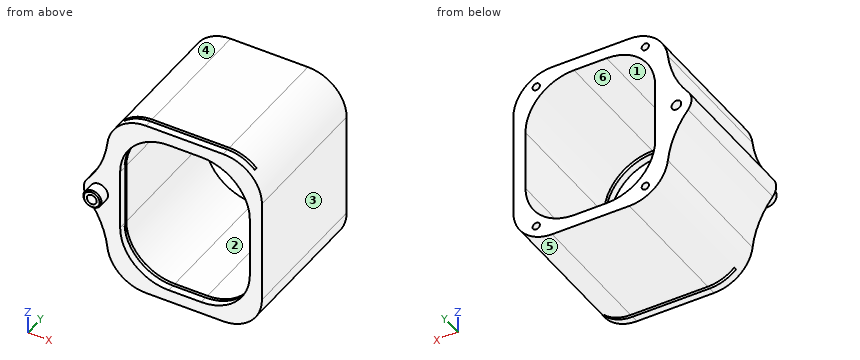
from build123d import *

# Parameters (mm, degrees)
CUT_EXTRUDE1_REACH       = 130.224
SKETCH3_W                = 13.598117377
SKETCH3_H                = 26.0138757
BOSS_EXTRUDE1_DEPTH      = 75
BOSS_EXTRUDE1_DEPTH_BACK = 75
SKETCH2_W                = 127
SKETCH2_H                = 117
BOSS_EXTRUDE3_START      = -117
BOSS_EXTRUDE3_DEPTH      = 117
CUT_EXTRUDE2_DEPTH       = 200.610245228
CUT_EXTRUDE2_DEPTH_BACK  = 200.610245228
SKETCH5_W                = 107
SKETCH5_H                = 130
CUT_EXTRUDE3_DEPTH       = 239.158035766
CUT_EXTRUDE3_DEPTH_BACK  = 239.158035766
SKETCH6_W                = 108
SKETCH6_H                = 2.5
FILLET3_R                = 40
FILLET2_R                = 32
CHAMFER1_SIZE            = 1
SKETCH7_R                = 3
CUT_EXTRUDE4_DEPTH       = 8


with BuildPart() as part:
    # Sketch1 → Revolve1 (revolve)
    with BuildSketch(Plane.XY, mode=Mode.PRIVATE) as revolve1_sk:
        Polygon((4, 0), (4, 127), (12.5, 127), (12.5, 10), (7.5, 10), (7.5, 0), align=None)
    revolve(revolve1_sk.sketch.rotate(Axis((0, 0, 0), (0, 1, 0)), 90), axis=Axis((0, 0, 0), (0, 1, 0)))

    # Sketch3 → Cut-Extrude1 (cut, up to next)
    with BuildSketch(Plane.XZ, mode=Mode.PRIVATE) as cut_extrude1_sk1:
        with Locations((14.299058689, 0)):
            Rectangle(SKETCH3_W, SKETCH3_H)
    cut_extrude1_tool1 = extrude(cut_extrude1_sk1.sketch, amount=-CUT_EXTRUDE1_REACH, mode=Mode.PRIVATE) & part.part
    add(cut_extrude1_tool1.solids().sort_by_distance((14.299059, 0, 0))[0], mode=Mode.SUBTRACT)



with BuildPart() as body_2:
    # Sketch2 → Boss-Extrude1 (new, two sides: drawn at the far end of the back side and taken through both)
    with BuildSketch(Plane.XY.offset(-BOSS_EXTRUDE1_DEPTH_BACK)):
        with Locations((71, 68.5)):
            Rectangle(SKETCH2_W, SKETCH2_H)
    extrude(amount=BOSS_EXTRUDE1_DEPTH + BOSS_EXTRUDE1_DEPTH_BACK)


with BuildPart() as part_1:
    add(part.part)

    add(body_2.part)  # Boss-Extrude3 merges body 2
    # Sketch4 → Boss-Extrude3 (add)
    with BuildSketch(Plane(origin=(0, 127, 0), x_dir=(1, 0, 0), z_dir=(0, 1, 0)).offset(BOSS_EXTRUDE3_START)):
        with BuildLine():
            Line((7.5, -55.677643628), (7.5, -10))
            ThreePointArc((7.5, -10), (-1.481398078, -12.411907981), (-9.642857143, -7.95394909))
            ThreePointArc((-9.642857143, -7.95394909), (3.084296109, -30.323015986), (7.5, -55.677643628))
        make_face()
        with BuildLine():
            Line((7.5, 10), (7.5, 55.677643628))
            ThreePointArc((7.5, 55.677643628), (3.084296109, 30.323015986), (-9.642857143, 7.95394909))
            ThreePointArc((-9.642857143, 7.95394909), (-1.481398078, 12.411907981), (7.5, 10))
        make_face()
    extrude(amount=BOSS_EXTRUDE3_DEPTH)

    # Sketch5 → Cut-Extrude2 (cut, two sides: drawn at the far end of the back side and taken through both)
    with BuildSketch(Plane(origin=(0, 127, 0), x_dir=(1, 0, 0), z_dir=(0, 1, 0)).offset(-CUT_EXTRUDE2_DEPTH_BACK)):
        with Locations((71, 0)):
            Rectangle(SKETCH5_W, SKETCH5_H)
    extrude(amount=CUT_EXTRUDE2_DEPTH + CUT_EXTRUDE2_DEPTH_BACK, mode=Mode.SUBTRACT)

    # Sketch6 → Cut-Extrude3 (cut, two sides: drawn at the far end of the back side and taken through both)
    with BuildSketch(Plane.XY.offset(75).offset(-CUT_EXTRUDE3_DEPTH_BACK)):
        with Locations((71, 17.25)):
            Rectangle(SKETCH6_W, SKETCH6_H)
    extrude(amount=CUT_EXTRUDE3_DEPTH + CUT_EXTRUDE3_DEPTH_BACK, mode=Mode.SUBTRACT)

    # Fillet3
    fillet3_edges = [part_1.edges().sort_by_distance(p)[0] for p in [
        (17.5, 13, -65),
        (124.5, 13, -65),
        (124.5, 13, 65),
        (17.5, 13, 65),
        (17.5, 72.75, -65),
        (17.5, 72.75, 65),
        (124.5, 72.75, 65),
        (124.5, 72.75, -65),
    ]]
    fillet(fillet3_edges, radius=FILLET3_R)

    # Fillet2
    # the kernel refuses this fillet: 32 mm, written as the material it takes off along each edge
    with BuildSketch(Plane(origin=(7.5, -68.115762804, -75), x_dir=(1, 0, 0), z_dir=(0, 1, 0))) as fillet2_piece_1:
        with BuildLine():
            CenterArc((31.246305122, -32), FILLET2_R, 90, 83.19545987)
            Line((-0.528290802, -28.208555177), (-3.705750395, -27.829410694))
            ThreePointArc((-3.705750395, -27.829410694), (-3.2, -19.322356372), (-3.2, 0))
            Line((-3.2, 0), (0, 3.2))
            Line((0, 3.2), (31.246305122, 3.2))
            Line((31.246305122, 3.2), (31.246305122, 0))
        make_face()
    extrude(amount=273.231525609, mode=Mode.SUBTRACT)
    with BuildSketch(Plane(origin=(134.5, 207, -75), x_dir=(0, 0, 1), z_dir=(0, -1, 0)), Plane(origin=(134.5, 207, 75), x_dir=(-1, 0, 0), z_dir=(0, -1, 0))) as fillet2_piece_2:
        with BuildLine():
            CenterArc((FILLET2_R, FILLET2_R), FILLET2_R, 180, 90)
            Line((0, FILLET2_R), (0, 0))
            Line((0, 0), (FILLET2_R, 0))
        make_face()
    extrude(amount=277, mode=Mode.SUBTRACT)
    with BuildSketch(Plane(origin=(7.5, -68.115762804, 75), x_dir=(1, 0, 0), z_dir=(0, 1, 0))) as fillet2_piece_3:
        with BuildLine():
            CenterArc((31.246305122, 32), FILLET2_R, 186.80454013, 83.19545987)
            Line((-0.528290802, 28.208555177), (-3.705750395, 27.829410694))
            ThreePointArc((-3.705750395, 27.829410694), (-3.2, 19.322356372), (-3.2, 0))
            Line((-3.2, 0), (0, -3.2))
            Line((0, -3.2), (31.246305122, -3.2))
            Line((31.246305122, -3.2), (31.246305122, 0))
        make_face()
    extrude(amount=273.231525609, mode=Mode.SUBTRACT)

    # Chamfer1
    chamfer1_edges = [part_1.edges().sort_by_distance(p)[0] for p in [
        (0, 0, 7.5),
    ]]
    chamfer(chamfer1_edges, length=CHAMFER1_SIZE)

    # Sketch7 → Cut-Extrude4 (cut)
    with BuildSketch(Plane(origin=(0, 127, 0), x_dir=(1, 0, 0), z_dir=(0, 1, 0))):
        with Locations(Location((115.623152561, -62.5, 0), (0, 0, 270))):
            Circle(SKETCH7_R)
        with Locations(Location((25.623152561, -62.5, 0), (0, 0, 270))):
            Circle(SKETCH7_R)
        with Locations(Location((25.623152561, 62.5, 0), (0, 0, 270))):
            Circle(SKETCH7_R)
        with Locations(Location((115.623152561, 62.5, 0), (0, 0, 270))):
            Circle(SKETCH7_R)
    extrude(amount=-CUT_EXTRUDE4_DEPTH, mode=Mode.SUBTRACT)


solid = part_1.part
Design review of the part built by this model. Coordinates are the model's own, in mm. Face numbers are marked on the shaded views. A direction names the side the tool comes from. Coordinates: 2 decimals unless noted, no trailing zeros. Write each loop counter-clockwise with the first axis right and the second up, starting at its lowest first coordinate (ties: lowest second). Pieces come first, ordered by that corner, then holes. Notation, with made-up numbers: (79, -1) - (117, -1) arc R26 cw to (117, 26) - close; hole circle Ø1 at (14.5, 15). An arc over 180 degrees is marked (long way). One line per item, written item: value.
1) Add section A-A (z = 0). State the section outline as (x, y) points.
Answer sheet:
outline: (-12.5, 10) - (-7.5, 10) - (-7.5, 1) - (-6.5, 0) - (-4, 0) - (-4, 127) - (-12.5, 127) - close; (4, 0) - (6.5, 0) - (7.5, 1) - (7.5, 10) - (17.5, 10) - (17.5, 16) - (17, 16) - (17, 18.5) - (17.5, 18.5) - (17.5, 127) - (4, 127) - close; (124.5, 10) - (134.5, 10) - (134.5, 127) - (124.5, 127) - (124.5, 18.5) - (125, 18.5) - (125, 16) - (124.5, 16) - close
2) For the marked faces 5 and 6, list the 3-axis set-ups (+Z, -Z, +X, -X, +Y, -Y) from which the entire face can be reached by the end or side of a thin tool; tool diameter is ignored.
Answer sheet:
face 5: -Z, +X, +Y, -Y
face 6: +Y, -Y
3) Add section B-B (z = -34). State the section outline as (x, y) points, plus the area to 3 significant figures.
Answer sheet:
outline: (4.3, 10) - (18.53, 10) - (18.53, 16) - (17, 16) - (17, 18.5) - (18.53, 18.5) - (18.53, 127) - (4.3, 127) - close; (123.47, 10) - (134.5, 10) - (134.5, 127) - (123.47, 127) - (123.47, 18.5) - (125, 18.5) - (125, 16) - (123.47, 16) - close
area: 2,950 mm2
4) Add section C-C (x = 91.5). State the section outline as (y, z) points.
Answer sheet:
outline: (10, -75) - (16, -75) - (16, -64.38) - (10, -64.38) - close; (10, 64.38) - (16, 64.38) - (16, 75) - (10, 75) - close; (18.5, -75) - (127, -75) - (127, -64.38) - (18.5, -64.38) - close; (18.5, 64.38) - (127, 64.38) - (127, 75) - (18.5, 75) - close
5) Mouldability with a two-part tool opening along Z and no side actions: class the marked faces 1, 2, 3 and 4 as +Z half, -Z half, draft (parallel to the pull), parting line (faces both ways), or undercut.
Answer sheet:
face 1: undercut
face 2: undercut
face 3: draft
face 4: +Z half
6) Add section D-D (y = 62). State the section outline as (x, z) points, plus the area to 3 significant figures.
Answer sheet:
outline: (-9.64, -7.95) arc R75 cw to (6.97, -46.79) arc R32 ccw to (38.75, -75) - (102.5, -75) arc R32 ccw to (134.5, -43) - (134.5, 43) arc R32 ccw to (102.5, 75) - (38.75, 75) arc R32 ccw to (6.97, 46.79) arc R75 cw to (-9.64, 7.95) arc R12.5 ccw to start; hole circle Ø8 at (0, 0); hole (17.5, -25) arc R40 ccw to (57.5, -65) - (84.5, -65) arc R40 ccw to (124.5, -25) - (124.5, 25) arc R40 ccw to (84.5, 65) - (57.5, 65) arc R40 ccw to (17.5, 25) - close
area: 6,450 mm2
7) To check wall thickness, follow probe 1 along X at (y, z) = (121, -62); probe 2 along Y at (x, z) = (117, 57); probe 3 along Z at (x, y) = (54, 36.5). State the ranges of each line that lie inside material, in increasing order.
Answer sheet:
probe 1: x = 13 to 22.67, 28.58 to 42.3, 99.7 to 112.67, 118.58 to 128.25
probe 2: y = 10 to 16, 18.5 to 127
probe 3: z = -75 to -64.85, 64.85 to 75
8) Insertion check: pin 1 (5 mm diameter, centred on x = 25, z = 61.5, fed in from +Y); pin 2 (3.5 mm diameter, centred on x = 115.62, z = 62.5, fed in from -Y); pin 3 (6 mm diameter, centred on y = 34, z = 18.5, fed in from -X); pin 4 (6 mm diameter, centred on y = 94, z = -36.5, fed in from -X). Each pin has a flat end and moves straight along its axis. Give the tip position at first contact, or say it passes through.
Answer sheet:
pin 1: stops at y = 127
pin 2: stops at y = 10
pin 3: stops at x = -4.17
pin 4: stops at x = 4.15
